Design review of the part built by this model. Coordinates are the model's own, in mm. A direction names the side the tool comes from. Round coordinates to 2 decimals unless told otherwise and drop trailing zeros. Loops run counter-clockwise (first coordinate to the right, second up) from the corner with the lowest first, then second, coordinate; pieces in that order, holes last. Notation, with made-up numbers: M 47.5,-15 L 89.5,-15 A22 cw 89.5,13 Z; hole C -25,56 d10. An arc over 180 degrees is marked long. Use a Markdown table: item, result.
from build123d import *
from OCP.BRepFilletAPI import BRepFilletAPI_MakeChamfer

# Parameters (mm, degrees)
SKETCH1_R           = 2.8
BOSS_EXTRUDE1_DEPTH = 1
BOSS_EXTRUDE2_DEPTH = 0.35
FILLET1_R           = 1.5
SKETCH3_W           = 1.3
SKETCH3_H           = 2
BOSS_EXTRUDE3_DEPTH = 0.7
CHAMFER1_SIZE       = 0.5
CHAMFER1_SIZE2      = 1.866025404
FILLET2_R           = 0.5
FILLET3_R           = 0.25
SHELL3_START        = -4.45
SHELL3_DEPTH        = 0.6
SHELL3_START_2      = 3.85
SHELL3_2_DEPTH      = 0.6


# Read off the part's stored shape, not the designer's step: Shell3
with BuildPart() as part:
    # Sketch1 → Boss-Extrude1 (new body)
    with BuildSketch(Plane(origin=(0, 0, 0), x_dir=(0, 0, -1), z_dir=(1, 0, 0))):
        Circle(SKETCH1_R)
    extrude(amount=BOSS_EXTRUDE1_DEPTH)

    # Sketch2 → Boss-Extrude2 (add)
    with BuildSketch(Plane(origin=(0, 0, 0), x_dir=(0, 0, -1), z_dir=(1, 0, 0))):
        with BuildLine():
            Line((2.5, -4.6), (5, -4.6))
            Line((5, -4.6), (5, 2.495381949))
            Line((5, 2.495381949), (5, 2.884339454))
            ThreePointArc((5, 2.884339454), (0, 4), (-5, 2.884339454))
            Line((-5, 2.884339454), (-5, 2.495381949))
            Line((-5, 2.495381949), (-5, -4.6))
            Line((-5, -4.6), (-2.5, -4.6))
            Line((-2.5, -4.6), (-2.5, -3.1))
            Line((-2.5, -3.1), (2.5, -3.1))
            Line((2.5, -3.1), (2.5, -4.6))
        make_face()
    extrude(amount=-BOSS_EXTRUDE2_DEPTH)

    # Fillet1
    # the kernel refuses this fillet: 1.5 mm, written as the material it takes off along each edge
    with BuildSketch(Plane(origin=(1, 0, 0), x_dir=(0, 0, -1), z_dir=(0, -1, 0))) as fillet1_piece_1:
        with BuildLine():
            CenterArc((1.385786438, -1.5), FILLET1_R, 19.471220634, 70.528779366)
            Line((1.385786438, 0), (1.385786438, 0.03))
            Line((1.385786438, 0.03), (2.8, 0.03))
            Line((2.8, 0.03), (2.83, 0))
            ThreePointArc((2.83, 0), (2.83, -0.5), (2.828284271, -0.99))
            Line((2.828284271, -0.99), (2.8, -1))
        make_face()
    revolve(axis=Axis((1, 0, 0), (1, 0, 0)), mode=Mode.SUBTRACT)

    # Sketch3 → Boss-Extrude3 (add)
    with BuildSketch(Plane(origin=(0, 0, 0), x_dir=(0, 0, -1), z_dir=(1, 0, 0))):
        with Locations((-4.15, 0)):
            Rectangle(SKETCH3_W, SKETCH3_H)
        with Locations((4.15, 0)):
            Rectangle(SKETCH3_W, SKETCH3_H)
    extrude(amount=BOSS_EXTRUDE3_DEPTH)

    # Chamfer1: one chamfer whose edges measure the first distance from different faces: ONE call of the kernel's chamfer builder (chamfer() names one face for all edges)
    chamfer1_edges_1 = [part.edges().sort_by_distance(p)[0] for p in [
        (0.7, -1, 4.15),
    ]]
    chamfer1_side_1 = [part.faces().sort_by_distance(p)[0] for p in [
        (0.35, -1, 4.15),
    ]]
    chamfer1_edges_2 = [part.edges().sort_by_distance(p)[0] for p in [
        (0.7, -1, -4.15),
    ]]
    chamfer1_side_2 = [part.faces().sort_by_distance(p)[0] for p in [
        (0.35, -1, -4.15),
    ]]
    chamfer1 = BRepFilletAPI_MakeChamfer(part.part.solid().wrapped)
    for e in chamfer1_edges_1:
        chamfer1.Add(CHAMFER1_SIZE, CHAMFER1_SIZE2, e.wrapped, chamfer1_side_1[0].wrapped)  # the first distance lies on this face
    for e in chamfer1_edges_2:
        chamfer1.Add(CHAMFER1_SIZE, CHAMFER1_SIZE2, e.wrapped, chamfer1_side_2[0].wrapped)  # the first distance lies on this face
    add(Compound.cast(chamfer1.Shape()), mode=Mode.REPLACE)

    # Fillet2
    fillet2_edges = [part.edges().sort_by_distance(p)[0] for p in [
        (-0.175, -3.1, 2.5),
        (-0.175, -3.1, -2.5),
    ]]
    fillet(fillet2_edges, radius=FILLET2_R)

    # Fillet3
    fillet3_edges = [part.edges().sort_by_distance(p)[0] for p in [
        (-0.175, -4.6, 2.5),
        (-0.175, -4.6, 5),
        (-0.175, 2.884339454, 5),
        (-0.175, 2.884339454, -5),
        (-0.175, -4.6, -5),
        (-0.175, -4.6, -2.5),
    ]]
    fillet(fillet3_edges, radius=FILLET3_R)

    # Shell3 outline → Shell3 (cut)
    with BuildSketch(Plane.XY.offset(SHELL3_START)):
        Polygon((-0.35, -0.65), (-0.068564446, -0.65), (0.279769504, 0.65), (-0.35, 0.65), align=None)
    extrude(amount=SHELL3_DEPTH, mode=Mode.SUBTRACT)

    # Shell3 2 outline → Shell3 2 (cut)
    with BuildSketch(Plane.XY.offset(SHELL3_START_2)):
        Polygon((-0.35, -0.65), (-0.068564446, -0.65), (0.279769504, 0.65), (-0.35, 0.65), align=None)
    extrude(amount=SHELL3_2_DEPTH, mode=Mode.SUBTRACT)

    # Shell3 3 outline → Shell3 3 (revolve, cut)
    with BuildSketch(Plane.YX):
        with BuildLine():
            ThreePointArc((2.525961863, -0.35), (2.144073982, 0.364580823), (1.385786438, 0.65))
            Line((1.385786438, 0.65), (0, 0.65))
            Line((0, 0.65), (0, -0.35))
            Line((0, -0.35), (2.525961863, -0.35))
        make_face()
    revolve(axis=Axis((0, 0, 0), (1, 0, 0)), mode=Mode.SUBTRACT)


solid = part.part
1. Take a section at A-A on x = -0.2. Give the boundary of the cut face in (y, z).
Check values:
| item | result |
|---|---|
| outline | M -4.6,-4.75 A0.25 ccw -4.35,-5 L 2.72,-5 A0.25 ccw 2.95,-4.85 A11.76 ccw 2.95,4.85 A0.25 ccw 2.72,5 L -4.35,5 A0.25 ccw -4.6,4.75 L -4.6,2.75 A0.25 ccw -4.35,2.5 L -3.6,2.5 A0.5 cw -3.1,2 L -3.1,-2 A0.5 cw -3.6,-2.5 L -4.35,-2.5 A0.25 ccw -4.6,-2.75 Z; hole C 0,0 d4.99; hole M -0.65,-4.45 L 0.65,-4.45 L 0.65,-3.85 L -0.65,-3.85 Z; hole M -0.65,3.85 L 0.65,3.85 L 0.65,4.45 L -0.65,4.45 Z |
2. Machinability: for faces 1 (the face through (0, 3, 1)), 2 (the face through (1, 0, 0)), 3 (the face through (0.453, -0.054, 4.159)), which of the approach directions +Z, -Z, +X, -X, +Y, -Y give a long, thin tool a straight path to every point of the face, cutting with its end or side? Answer none if there is none.
Check values:
| item | result |
|---|---|
| face 1 | +X |
| face 2 | +Z, -Z, +X, +Y, -Y |
| face 3 | +Z, +X, -Y |
3. Take a section at B-B on x = 0.4. Count the separate pieces of the cut face and the enclosed holes in it, and give its area (3 significant figures).
Check values:
| item | result |
|---|---|
| separate pieces | 3 |
| enclosed holes | 1 |
| area | 10.4 mm² |
4. Insertion check: pin 1 (0.8 mm diameter, centred on y = -0.5, z = 0.5, fed in from -X); pin 2 (0.8 mm diameter, centred on x = 0.5, y = -0.5, fed in from -Z). Each pin has a flat end and moves straight along its axis. Give the tip position at first contact, or say it passes through.
Check values:
| item | result |
|---|---|
| pin 1 | stops at x = 0.65 |
| pin 2 | stops at z = -4.8 |
5. Wall thickness on line 1 along X through (y, z) = (-2, -2); line 2 along Y through (x, z) = (-0.15, 1.5); line 3 along Z through (x, y) = (0.1, 1.75) (3 decimals): over which ranges is each line inside the solid? List them lowest first. Write a range as from..to.
Check values:
| item | result |
|---|---|
| line 1 | x = -0.35..0 |
| line 2 | y = -3.1..-1.98, 1.98..3.9 |
| line 3 | z = -2.135..-1.594, 1.594..2.135 |
6. The part is to be moulded in two halves that separate along Z. For faces 4 (the face through (0.453, -0.054, -4.141)), 5 (the face through (-0.2, 4, -0.1)), 6 (the face through (0.65, 0, 0)), say which applies: pulls with the +Z half, pulls with the -Z half, needs draft (parallel to the pull), parting line crosses it, or undercut.
Check values:
| item | result |
|---|---|
| face 4 | needs draft |
| face 5 | parting line crosses it |
| face 6 | undercut |
